```python
from build123d import *

# Parameters (mm, degrees)
CYLINDER001_R     = 3
CYLINDER001_DEPTH = 9
CYLINDER_R        = 2.2
CYLINDER_DEPTH    = 9
SKETCH_R          = 18
PAD_DEPTH         = 25
SKETCH001_R       = 13
SKETCH001_R_2     = 5
POCKET_DEPTH      = 10
SKETCH002_R       = 13
POCKET001_DEPTH   = 12
SKETCH003_R       = 1.6
POCKET002_DEPTH   = 13
FILLET_R          = 3


with BuildPart() as cilindro001:
    # Cylinder001 → Cylinder001 (new body)
    with BuildSketch(Plane(origin=(0, 20, 21), x_dir=(1, 0, 0), z_dir=(0, -1, 0))):
        Circle(CYLINDER001_R)
    extrude(amount=CYLINDER001_DEPTH)


with BuildPart() as cilindro:
    # Cylinder → Cylinder (new body)
    with BuildSketch(Plane(origin=(0, 9, 21), x_dir=(1, 0, 0), z_dir=(0, -1, 0))):
        Circle(CYLINDER_R)
    extrude(amount=CYLINDER_DEPTH)


with BuildPart() as cut001:
    # Sketch → Pad (new body)
    with BuildSketch(Plane.XY):
        Circle(SKETCH_R)
    extrude(amount=PAD_DEPTH)

    # Sketch001 (on Face3 of Pad) → Pocket (cut)
    with BuildSketch(Plane.XY.offset(25)):
        Circle(SKETCH001_R)
        Circle(SKETCH001_R_2, mode=Mode.SUBTRACT)
    extrude(amount=-POCKET_DEPTH, mode=Mode.SUBTRACT)

    # Sketch002 (on Face2 of Pocket) → Pocket001 (cut)
    with BuildSketch(Plane(origin=(0, 0, 0), x_dir=(1, 0, 0), z_dir=(0, 0, -1))):
        Circle(SKETCH002_R)
    extrude(amount=-POCKET001_DEPTH, mode=Mode.SUBTRACT)

    # Sketch003 (on Face9 of Pocket001) → Pocket002 (cut)
    with BuildSketch(Plane.XY.offset(25)):
        Circle(SKETCH003_R)
    extrude(amount=-POCKET002_DEPTH, mode=Mode.SUBTRACT)

    # Fillet
    fillet_edges = [cut001.edges().sort_by_distance(p)[0] for p in [
        (-5, 0, 15),
        (-13, 0, 15),
        (-13, 0, 12),
    ]]
    fillet(fillet_edges, radius=FILLET_R)

    # Cut: cut Cilindro
    add(cilindro.part, mode=Mode.SUBTRACT)

    # Cut001: cut Cilindro001
    add(cilindro001.part, mode=Mode.SUBTRACT)


solid = cut001.part
```
Design review of the part built by this model. Coordinates are the model's own, in mm. A direction names the side the tool comes from. Coordinates: 2 decimals unless noted, no trailing zeros. Order: outer loops, then holes, each group sorted by start corner. A loop starts at its lowest first (then second) coordinate and runs counter-clockwise, first axis right, second up. Notation, with made-up numbers: M 8,-15.75 L 25,-15.75 A26 ccw 25,9.25 Z; hole C -0.5,51 d6. An arc over 180 degrees is marked long. Answer as a JSON object with one key per item and string values. Group by question number.
1) Add section A-A, the plane z = 21.75. Write out the cut boundary in (x, y).
2) Tool access review of faces 1 (the cylindrical face through (-2.198, 2.537, 21.097)), 2 (the cylindrical face through (-3.902, -17.572, 12.325)), 3 (the cylindrical face through (-2.82, -12.69, 21.55)): name each direction out of +Z, -Z, +X, -X, +Y, -Y from which nothing blocks a thin tool from reaching the whole face with its end or side.
3) Add section D-D, the plane x = -16. Write out the cut boundary in (y, z).
4) Wall thickness on L1, parallel to Y at x = 0, z = 23.5; L2, parallel to Z at x = 0, y = 3; L3, parallel to Y at x = 0, z = 20: over which ranges is each line inside the solid? List them lowest first.
5) Add section B-B, the plane z = 7. Write out the cut boundary in (x, y).
6) Mouldability with a two-part tool opening along Z and no side actions: class faces 4 (the cylindrical face through (2.77, 15.36, 19.85)), 5 (the flat face through (2, 0, 12)), 6 (the flat face through (0, 8.2, 15)), 7 (the cylindrical face through (-10.316, 7.91, 4.437)) as pulls with the +Z half, pulls with the -Z half, needs draft (parallel to the pull), parting line crosses it, or undercut.
7) Add section C-C, the plane y = -13.5. Write out the cut boundary in (x, z).
8) For pin 1 (3 mm diameter, centred on x = 5.5, z = 6.5, fed in from +Y); pin 2 (0.7 mm diameter, centred on x = 2, z = 21.5, fed in from +Y); pin 3 (6 mm diameter, centred on x = 5.5, z = 8, fed in from +Y), all flat-tipped, find the tip position at first contact; note any pin that passes through.
Computed values:
{
 "1": {"outline": "M -2.9,12.67 L -2.9,17.76 A18 ccw long 2.9,17.76 L 2.9,12.67 A13 cw long Z; M -2.07,0 L -2.07,4.55 A5 ccw long 2.07,4.55 L 2.07,0 L 1.6,0 A1.6 cw -1.6,0 Z"},
 "2": {"face 1": "+Y", "face 2": "+Z, -Z", "face 3": "+Z"},
 "3": {"outline": "M -8.25,0 L 8.25,0 L 8.25,25 L -8.25,25 Z"},
 "4": {"L1": "y = -18 to -13, -5 to -1.6, 1.6 to 5", "L2": "z = 12 to 18.8, 23.2 to 25", "L3": "y = -18 to -13, -5 to -1.6"},
 "5": {"outline": "C 0,0 d36; hole C 0,0 d26"},
 "6": {"face 4": "undercut", "face 5": "pulls with the -Z half", "face 6": "pulls with the +Z half", "face 7": "needs draft"},
 "7": {"outline": "M -11.91,0 L 11.91,0 L 11.91,25 L -11.91,25 Z"},
 "8": {"pin 1": "stops at y = 17.55", "pin 2": "stops at y = 4.57", "pin 3": "stops at y = 17.83"}
}
